Read the model definition and answer for the solid it produces. Units are mm, in the model's axes. A direction names the side the tool comes from. Round coordinates to 2 decimals unless told otherwise and drop trailing zeros. Loops run counter-clockwise (first coordinate to the right, second up) from the corner with the lowest first, then second, coordinate; pieces in that order, holes last. Notation, with made-up numbers: (-20, 55) - (29, 55) arc R20 ccw to (29, 80) - close; hole circle Ø6 at (66.25, 80). An arc over 180 degrees is marked (long way). Use CSV: the item, a comma, the result in double quotes. Start each with the question number.
1. Consider line 1 along Y through (x, z) = (46, 25); line 2 along X through (y, z) = (40.5, 17); line 3 along X through (y, z) = (-16, 35). Determine where each line is inside the solid, lowest interval first.
2. Given pin 1 Ø9.5 at (y, z) = (-22, 34.5) entering from +X; pin 2 Ø12 at (x, z) = (96, 11) entering from -Y; pin 3 Ø16.5 at (x, y) = (70, -18) entering from -Z, each flat-ended and moving along its own axis, determine where each tip first touches the part or whether it passes through.
3. Find section B-B (y = 51.5). Give the vertices of the cut face in (x, z).
4. Find section C-C (z = 8). Give the vertices of the cut face in (x, y).
5. Determine the mould class of faces 5 (the flat face through (31.79, 47, 19)), 6 (the flat face through (0, 34, 19)), 7 (the flat face through (71, -15, 26.528)), 8 (the flat face through (44, 53.144, 19)) for opening direction X: +X half, -X half, draft (parallel to the pull), parting line (faces both ways), or undercut.
6. Find section D-D (x = 71.12). Give the vertices of the cut face in (y, z).
7. A tool of negligible diameter and unlimited length cuts with its end or side. For faces 1 (the flat face through (63.592, -16, 32)), 2 (the flat face through (78.648, -15, 32)), 3 (the flat face through (98, 53.144, 19)), 4 (the flat face through (57.19, 60, 19)), from which of +Z, -Z, +X, -X, +Y, -Y can it reach the whole face along a straight path? Write none if from no direction.
8. Find section A-A (x = 101). Give the vertices of the cut face in (y, z).
from build123d import *

# Parameters (mm, degrees)
BOSS_EXTRUDE1_DEPTH = 38.1
SKETCH2_R           = 8.7503
BOSS_EXTRUDE2_DEPTH = 38.1
BOSS_EXTRUDE6_DEPTH = 11.572281197


with BuildPart() as part:
    # Sketch1 → Boss-Extrude1 (new body)
    with BuildSketch(Plane.XY):
        Polygon((0, 0), (142.319474343, 0), (142.319474343, 67.883016851), (85.129737171, 67.883016851), (85.129737171, 53.144138708), (110.529737171, 53.144138708), (110.529737171, 40.190138708), (31.789737171, 40.190138708), (31.789737171, 53.144138708), (57.189737171, 53.144138708), (57.189737171, 67.883016851), (0, 67.883016851), align=None)
    extrude(amount=BOSS_EXTRUDE1_DEPTH)



with BuildPart() as body_2:
    # Sketch2 → Boss-Extrude2 (new body)
    with BuildSketch(Plane.XY.offset(38.1)):
        with Locations((71.120000025, -35.559977798)):
            Circle(SKETCH2_R)
    extrude(amount=-BOSS_EXTRUDE2_DEPTH)


with BuildPart() as part_1:
    add(part.part)

    add(body_2.part)  # Boss-Extrude6 merges body 2
    # Sketch8 → Boss-Extrude6 (add)
    with BuildSketch(Plane.XY.offset(38.1)):
        with BuildLine():
            Line((63.59200581, -40.020589099), (63.59200581, 0))
            Line((63.59200581, 0), (78.647994227, 0))
            Line((78.647994227, 0), (78.647994227, -40.020589121))
            ThreePointArc((78.647994227, -40.020589121), (71.120000012, -44.310277798), (63.59200581, -40.020589099))
        make_face()
    extrude(amount=-BOSS_EXTRUDE6_DEPTH)


solid = part_1.part
Filled sheet:
1,line 1,"y = 0 to 40.19, 53.14 to 67.88"
1,line 2,"x = 0 to 31.79, 110.53 to 142.32"
1,line 3,"x = 63.59 to 78.65"
2,pin 1,"stops at x = 78.65"
2,pin 2,"stops at y = 0"
2,pin 3,"stops at z = 26.53"
3,outline,"(0, 0) - (31.79, 0) - (31.79, 38.1) - (0, 38.1) - close; (110.53, 0) - (142.32, 0) - (142.32, 38.1) - (110.53, 38.1) - close"
4,outline,"(0, 0) - (142.32, 0) - (142.32, 67.88) - (85.13, 67.88) - (85.13, 53.14) - (110.53, 53.14) - (110.53, 40.19) - (31.79, 40.19) - (31.79, 53.14) - (57.19, 53.14) - (57.19, 67.88) - (0, 67.88) - close; circle Ø17.5 at (71.12, -35.56)"
5,face 5,"undercut"
5,face 6,"-X half"
5,face 7,"draft"
5,face 8,"undercut"
6,outline,"(-44.31, 0) - (-26.81, 0) - (-26.81, 26.53) - (0, 26.53) - (0, 0) - (40.19, 0) - (40.19, 38.1) - (-44.31, 38.1) - close"
7,face 1,"+Z, -Z, -X"
7,face 2,"+Z, -Z, +X"
7,face 3,"+Z, -Z"
7,face 4,"+Z, -Z, +Y"
8,outline,"(0, 0) - (40.19, 0) - (40.19, 38.1) - (0, 38.1) - close; (53.14, 0) - (67.88, 0) - (67.88, 38.1) - (53.14, 38.1) - close"
